Check sheet for the modelled part. Datum: model origin and axes. Units: mm. A direction names the side the tool comes from. Give positions to 0.01 mm unless a question says otherwise; leave off trailing zeros. Write each loop counter-clockwise with the first axis right and the second up, starting at its lowest first coordinate (ties: lowest second). Pieces come first, ordered by that corner, then holes. Notation, with made-up numbers: (68, 28) -> (72, 28) arc R7 ccw to (72, 39) -> close; hole circle Ø8 at (-27, 80). An arc over 180 degrees is marked (long way). Use a Markdown table: item, result. Add a question column.
1. Release check for a two-part mould opening along Z. For faces 3 (the flat face through (-172.275, 3, -5)), 4 (the flat face through (-2, 3, -90.782)), 5 (the flat face through (-51, 2.3, -84)) record: released by +Z, released by -Z, zero draft, split by the parting line, or undercut.
2. Set-up check for faces 1 (the flat face through (-160.275, 3, -5)), 2 (the flat face through (-2, 3, 78.218)): record each of +Z, -Z, +X, -X, +Y, -Y from which the full face is reachable in a straight line by a thin tool's end or side.
3. Cross-section at C-C (x = -8). Enter the section's corners in (y, z), then the cut area to 3 significant figures.
4. Gauge pin test, flat ends, axial feed: P1, Ø2.5, axis at x = -165.5, z = 40, coming from the -Y side; P2, Ø0.8, axis at x = -90, z = -83.5, coming from the -Y side. Record the tip position at first contact, or that the pin passes through.
5. Cross-section at B-B (z = -11). Enter the section's corners in (x, y) (3 decimals).
6. Cross-section at A-A (x = -141). Enter the section's corners in (y, z), then the cut area to 3 significant figures.
7. Cross-section at D-D (z = 44). Enter the section's corners in (x, y) (3 decimals).
8. Scan lines: probe 1 along Z at (x, y) = (81, 3); probe 2 along X at (y, z) = (2.25, -73) (3 decimals); probe 3 along X at (y, z) = (1, -51) (3 decimals). Record each from-to range of solid material in increasing order. Write a range as [from, to].
from build123d import *

# Parameters (mm, degrees)
SKETCH1_W           = 344.55
SKETCH1_H           = 169
SKETCH1_W_2         = 320.55
SKETCH1_H_2         = 145
BOSS_EXTRUDE1_DEPTH = 7
FILLET1_R           = 5
FILLET2_R           = 5
FILLET3_R           = 5
CUT_EXTRUDE2_DEPTH  = 2.3
FILLET5_R           = 5
SKETCH4_R           = 1.325
CUT_EXTRUDE3_DEPTH  = 4


with BuildPart() as part:
    # Sketch1 → Boss-Extrude1 (new body)
    with BuildSketch(Plane(origin=(0, 0, 0), x_dir=(1, 0, 0), z_dir=(0, 1, 0))):
        with Locations((0, 6.282475928)):
            Rectangle(SKETCH1_W, SKETCH1_H)
        with Locations((0, 6.282475928)):
            Rectangle(SKETCH1_W_2, SKETCH1_H_2, mode=Mode.SUBTRACT)
    extrude(amount=BOSS_EXTRUDE1_DEPTH)

    # Fillet1
    fillet1_edges = [part.edges().sort_by_distance(p)[0] for p in [
        (172.275, 3.5, 78.217524072),
    ]]
    fillet(fillet1_edges, radius=FILLET1_R)

    # Fillet2
    fillet2_edges = [part.edges().sort_by_distance(p)[0] for p in [
        (-172.275, 3.5, -90.782475928),
    ]]
    fillet(fillet2_edges, radius=FILLET2_R)

    # Fillet3
    fillet3_edges = [part.edges().sort_by_distance(p)[0] for p in [
        (-172.275, 3.5, 78.217524072),
    ]]
    fillet(fillet3_edges, radius=FILLET3_R)

    # Sketch3 → Cut-Extrude2 (cut)
    with BuildSketch(Plane.XZ):
        Polygon((-22.72, -82.082475928), (-47.57, -82.082475928), (-47.57, -78.782475928), (-53.87, -78.782475928), (-53.87, -82.082475928), (-78.72, -82.082475928), (-78.72, -86.582475928), (-22.72, -86.582475928), align=None)
        Polygon((-130.175, 66.217524072), (-123.875, 66.217524072), (-123.875, 69.517524072), (-99.025, 69.517524072), (-99.025, 74.017524072), (-155.025, 74.017524072), (-155.025, 69.517524072), (-130.175, 69.517524072), align=None)
        Polygon((146.225, -82.082475928), (121.375, -82.082475928), (121.375, -78.782475928), (115.075, -78.782475928), (115.075, -82.082475928), (90.225, -82.082475928), (90.225, -86.582475928), (146.225, -86.582475928), align=None)
        Polygon((71.33, -86.582475928), (71.33, -82.082475928), (46.48, -82.082475928), (46.48, -78.782475928), (40.18, -78.782475928), (40.18, -82.082475928), (15.33, -82.082475928), (15.33, -86.582475928), align=None)
        Polygon((-160.275, -44.082475928), (-160.275, -50.382475928), (-163.575, -50.382475928), (-163.575, -75.232475928), (-168.075, -75.232475928), (-168.075, -19.232475928), (-163.575, -19.232475928), (-163.575, -44.082475928), align=None)
        Polygon((163.575, 11.917524072), (163.575, 32.217524072), (160.275, 32.217524072), (160.275, 38.517524072), (163.575, 38.517524072), (163.575, 58.817524072), (168.075, 58.817524072), (168.075, 11.917524072), align=None)
        Polygon((160.275, -40.582475928), (163.575, -40.582475928), (163.575, -15.732475928), (168.075, -15.732475928), (168.075, -71.732475928), (163.575, -71.732475928), (163.575, -46.882475928), (160.275, -46.882475928), align=None)
        Polygon((146.225, 74.017524072), (146.225, 69.517524072), (121.375, 69.517524072), (121.375, 66.217524072), (115.075, 66.217524072), (115.075, 69.517524072), (90.225, 69.517524072), (90.225, 74.017524072), align=None)
        Polygon((15.33, 74.017524072), (71.33, 74.017524072), (71.33, 69.517524072), (46.48, 69.517524072), (46.48, 66.217524072), (40.18, 66.217524072), (40.18, 69.517524072), (15.33, 69.517524072), align=None)
        Polygon((-160.275, 38.517524072), (-160.275, 32.217524072), (-163.575, 32.217524072), (-163.575, 11.917524072), (-168.075, 11.917524072), (-168.075, 58.817524072), (-163.575, 58.817524072), (-163.575, 38.517524072), align=None)
        Polygon((-55.375, 66.217524072), (-49.075, 66.217524072), (-49.075, 69.517524072), (-24.225, 69.517524072), (-24.225, 74.017524072), (-80.225, 74.017524072), (-80.225, 69.517524072), (-55.375, 69.517524072), align=None)
    extrude(amount=-CUT_EXTRUDE2_DEPTH, mode=Mode.SUBTRACT)

    # Fillet5
    fillet5_edges = [part.edges().sort_by_distance(p)[0] for p in [
        (172.275, 3.5, -90.782475928),
    ]]
    fillet(fillet5_edges, radius=FILLET5_R)

    # Sketch4 → Cut-Extrude3 (cut)
    with BuildSketch(Plane.XZ):
        with Locations(Location((-165.542766953, 71.485291024, 0), (0, 0, 270))):
            Circle(SKETCH4_R)
        with Locations(Location((-89.625, 71.767524072, 0), (0, 0, 270))):
            Circle(SKETCH4_R)
        with Locations(Location((80.7775, 71.767524072, 0), (0, 0, 270))):
            Circle(SKETCH4_R)
        with Locations(Location((165.532766953, 71.485291024, 0), (0, 0, 270))):
            Circle(SKETCH4_R)
        with Locations(Location((165.532766953, -84.050242881, 0), (0, 0, 270))):
            Circle(SKETCH4_R)
        with Locations(Location((80.7775, -84.332475928, 0), (0, 0, 270))):
            Circle(SKETCH4_R)
        with Locations(Location((-89.625, -84.050242881, 0), (0, 0, 270))):
            Circle(SKETCH4_R)
        with Locations(Location((-165.542766953, -84.050242881, 0), (0, 0, 270))):
            Circle(SKETCH4_R)
    extrude(amount=-CUT_EXTRUDE3_DEPTH, mode=Mode.SUBTRACT)


solid = part.part
Worked answers:
| question | item | result |
|---|---|---|
| 1 | face 3 | zero draft |
| 1 | face 4 | released by -Z |
| 1 | face 5 | undercut |
| 2 | face 1 | +Y, -Y |
| 2 | face 2 | +Z, +X, -X, +Y, -Y |
| 3 | outline | (0, -90.78) -> (7, -90.78) -> (7, -78.78) -> (0, -78.78) -> close; (0, 66.22) -> (7, 66.22) -> (7, 78.22) -> (0, 78.22) -> close |
| 3 | area | 168 mm² |
| 4 | P1 | stops at y = 2.3 |
| 4 | P2 | stops at y = 4 |
| 5 | outline | (-172.275, 0) -> (-160.275, 0) -> (-160.275, 7) -> (-172.275, 7) -> close; (160.275, 0) -> (172.275, 0) -> (172.275, 7) -> (160.275, 7) -> close |
| 6 | outline | (0, -90.78) -> (7, -90.78) -> (7, -78.78) -> (0, -78.78) -> close; (0, 66.22) -> (7, 66.22) -> (7, 78.22) -> (0, 78.22) -> (0, 74.02) -> (2.3, 74.02) -> (2.3, 69.52) -> (0, 69.52) -> close |
| 6 | area | 158 mm² |
| 7 | outline | (-172.275, 0) -> (-168.075, 0) -> (-168.075, 2.3) -> (-163.575, 2.3) -> (-163.575, 0) -> (-160.275, 0) -> (-160.275, 7) -> (-172.275, 7) -> close; (160.275, 0) -> (163.575, 0) -> (163.575, 2.3) -> (168.075, 2.3) -> (168.075, 0) -> (172.275, 0) -> (172.275, 7) -> (160.275, 7) -> close |
| 8 | probe 1 | z = [-90.78, -85.64], [-83.03, -78.78], [66.22, 70.46], [73.07, 78.22] |
| 8 | probe 2 | x = [-172.275, -168.075], [-163.575, -160.275], [160.275, 172.275] |
| 8 | probe 3 | x = [-172.275, -168.075], [-163.575, -160.275], [160.275, 163.575], [168.075, 172.275] |
